Can you work these out from the drawing? Everything is in mm from the part's minimum corner. Coordinates: 2 decimals unless noted, no trailing zeros. Loops run counter-clockwise (first coordinate to the right, second up) from the corner with the lowest first, then second, coordinate; pieces in that order, holes last.
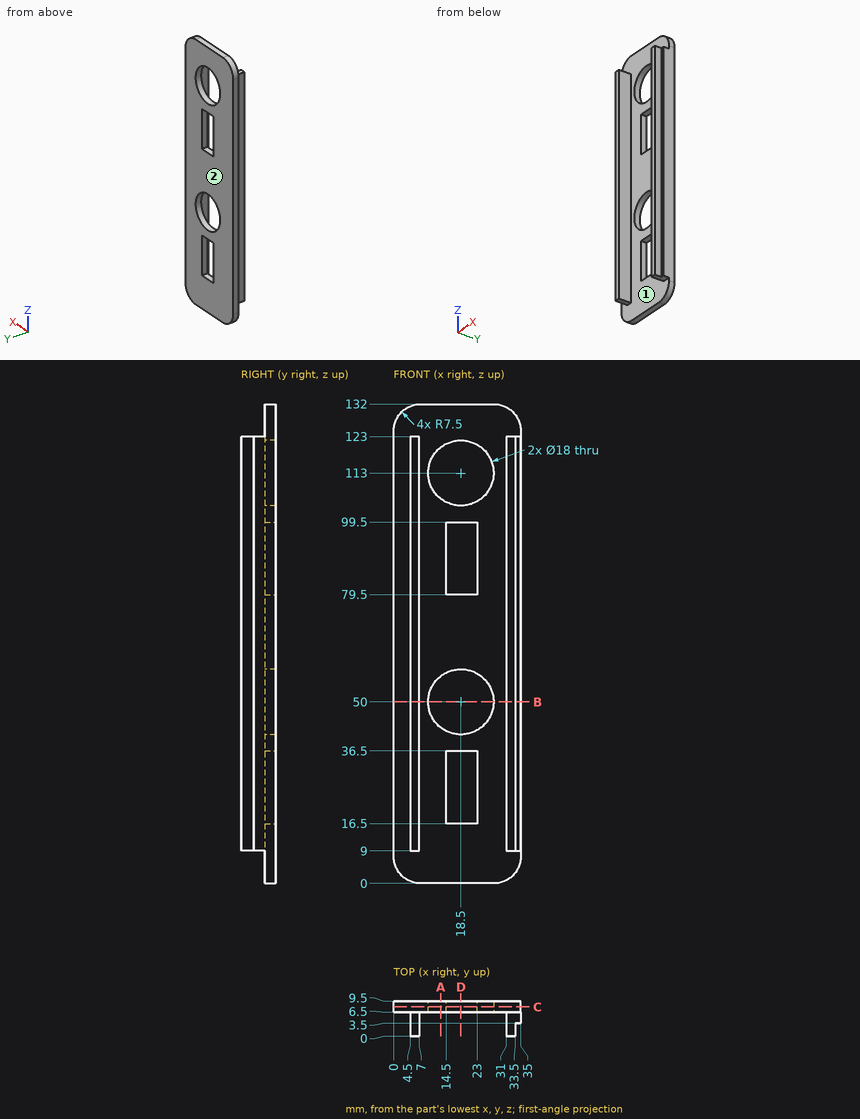
(1) For pin 1 (6 mm diameter, centred on x = 18.5, z = 106, fed in from -Y); pin 2 (2 mm diameter, centred on x = 5.5, y = 4, fed in from -Z); pin 3 (1 mm diameter, centred on y = 2, z = 42.5, fed in from +X), each with a flat end and sliding along its axis, tell me the tip position at first contact or that it passes through.
Answers:
pin 1: stops at y = 6.5
pin 2: stops at z = 9
pin 3: stops at x = 33.5
(2) Imagine slicing it at A-A, the plane x = 13. Write out the boundary of the cut face in (y, z).
Answers:
outline: (6.5, 0) - (9.5, 0) - (9.5, 42.88) - (6.5, 42.88) - close; (6.5, 57.12) - (9.5, 57.12) - (9.5, 105.88) - (6.5, 105.88) - close; (6.5, 120.12) - (9.5, 120.12) - (9.5, 132) - (6.5, 132) - close
(3) We'd pull the mould along X, two halves only. Please class the marked faces 1 and 2: +X half, -X half, draft (parallel to the pull), parting line (faces both ways), or undercut.
Answers:
face 1: undercut
face 2: draft
(4) Imagine slicing it at B-B, the plane z = 50. Write out the boundary of the cut face in (x, y).
Answers:
outline: (0, 6.5) - (4.5, 6.5) - (4.5, 0) - (7, 0) - (7, 6.5) - (9.5, 6.5) - (9.5, 9.5) - (0, 9.5) - close; (27.5, 6.5) - (31, 6.5) - (31, 0) - (33.5, 0) - (33.5, 3.5) - (35, 3.5) - (35, 9.5) - (27.5, 9.5) - close
(5) Imagine slicing it at D-D, the plane x = 18.5. Write out the boundary of the cut face in (y, z).
Answers:
outline: (6.5, 0) - (9.5, 0) - (9.5, 16.5) - (6.5, 16.5) - close; (6.5, 36.5) - (9.5, 36.5) - (9.5, 41) - (6.5, 41) - close; (6.5, 59) - (9.5, 59) - (9.5, 79.5) - (6.5, 79.5) - close; (6.5, 99.5) - (9.5, 99.5) - (9.5, 104) - (6.5, 104) - close; (6.5, 122) - (9.5, 122) - (9.5, 132) - (6.5, 132) - close
(6) I need wall thicknesses on probe 1 along Z at (x, y) = (18.5, 8.15); probe 2 along X at (y, z) = (6.25, 16); probe 3 along Z at (x, y) = (11, 9.25). Which ranges of each line are inside material? Lowest first, please.
Answers:
probe 1: z = 0 to 16.5, 36.5 to 41, 59 to 79.5, 99.5 to 104, 122 to 132
probe 2: x = 4.5 to 7, 31 to 35
probe 3: z = 0 to 45.03, 54.97 to 108.03, 117.97 to 132
(7) Imagine slicing it at C-C, the plane y = 8. Write out the boundary of the cut face in (x, z), and give its area (3 significant figures).
Answers:
outline: (0, 7.5) arc R7.5 ccw to (7.5, 0) - (27.5, 0) arc R7.5 ccw to (35, 7.5) - (35, 124.5) arc R7.5 ccw to (27.5, 132) - (7.5, 132) arc R7.5 ccw to (0, 124.5) - close; hole circle Ø18 at (18.5, 50); hole circle Ø18 at (18.5, 113); hole (14.5, 16.5) - (23, 16.5) - (23, 36.5) - (14.5, 36.5) - close; hole (14.5, 79.5) - (23, 79.5) - (23, 99.5) - (14.5, 99.5) - close
area: 3,720 mm2
